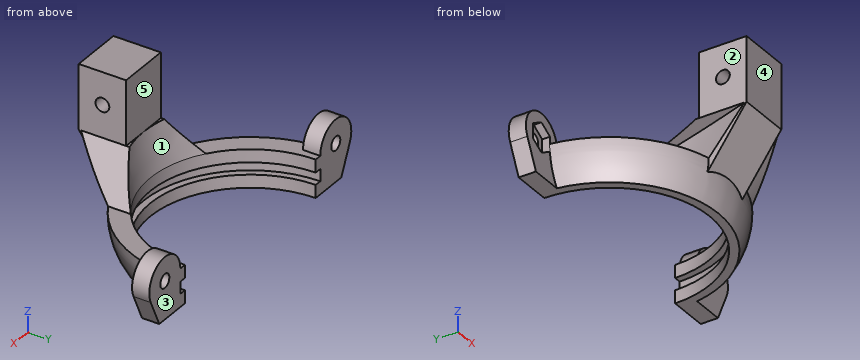
```python
from build123d import *

# Parameters (mm, degrees)
SKETCH005_R          = 1.6
PAD001_DEPTH         = 6.15
REVOLUTION_ANGLE     = -180
PAD_DEPTH            = 4
SKETCH002_R          = 1.6
POCKET_DEPTH         = 5
POCKET001_DEPTH      = 1.8
SKETCH004_R          = 3
POCKET002_DEPTH      = 2
REVOLUTION001_ANGLE  = 70
POCKET003_DEPTH      = 184.719613
POCKET003_DEPTH_BACK = 198.519612


with BuildPart() as pad001:
    # Sketch005 → Pad001 (new body, symmetric)
    with BuildSketch(Plane.YZ):
        Polygon((-35.8, 27.909628), (-24.8, 27.909628), (-24.8, -2.8), (-35.8, 12.909628), align=None)
        with Locations((-30.3, 20.409628)):
            Circle(SKETCH005_R, mode=Mode.SUBTRACT)
    extrude(amount=PAD001_DEPTH, both=True)


with BuildPart() as obj1:
    # Sketch → Revolution (revolve)
    with BuildSketch(Plane.XZ):
        with BuildLine():
            Line((23.2, 0), (24.8, 0))
            Line((24.8, 0), (24.8, -2.8))
            Line((24.8, -2.8), (23.2, -2.8))
            Line((23.2, -2.8), (23.2, -5.8))
            Line((23.2, -5.8), (25.2, -5.8))
            ThreePointArc((25.2, -5.8), (27.062874, -1.574112), (27.7, 3))
            Line((27.7, 3), (23.2, 3))
            Line((23.2, 0), (23.2, 3))
        make_face()
    revolve(axis=Axis((0, 0, 0), (0, 0, 1)), revolution_arc=REVOLUTION_ANGLE)

    # Sketch001 → Pad (new body)
    with BuildSketch(Plane(origin=(0, 0, 0), x_dir=(1, 0, 0), z_dir=(0, 1, 0))):
        with BuildLine():
            ThreePointArc((24.8, -3), (31.490407, -8.36963), (35.284703, -0.67562))
            Line((32.265071, 5.8), (35.284703, -0.67562))
            Line((24.8, 5.8), (32.265071, 5.8))
            Line((24.8, -3), (24.8, 5.8))
        make_face()
    pad = extrude(amount=-PAD_DEPTH)

    # Mirrored: Pad across Sketch001 V_Axis
    add(pad.mirror(Plane.YZ))

    # Sketch002 → Pocket (cut)
    with BuildSketch(Plane(origin=(0, 0, 0), x_dir=(1, 0, 0), z_dir=(0, 1, 0))):
        with Locations((-30.3, -3)):
            Circle(SKETCH002_R)
    pocket = extrude(amount=-POCKET_DEPTH, mode=Mode.SUBTRACT)

    # Mirrored001: Pocket across Sketch002 V_Axis
    add(pocket.mirror(Plane.YZ), mode=Mode.SUBTRACT)

    # Sketch003 → Pocket001 (cut)
    with BuildSketch(Plane.XZ.offset(4)):
        Polygon((-30.3, 6.464101), (-33.3, 4.73205), (-33.3, 1.267949), (-30.3, -0.464102), (-27.3, 1.267949), (-27.3, 4.73205), align=None)
    extrude(amount=-POCKET001_DEPTH, mode=Mode.SUBTRACT)

    # Sketch004 → Pocket002 (cut)
    with BuildSketch(Plane.XZ.offset(4)):
        with Locations((30.3, 3)):
            Circle(SKETCH004_R)
    extrude(amount=POCKET002_DEPTH, mode=Mode.SUBTRACT)

    # Fusion: union Pad001
    add(pad001.part)


with BuildPart() as mount_part:
    # Sketch006 → Revolution001 (revolve, symmetric)
    with BuildSketch(Plane.YZ) as revolution001_sk:
        Polygon((-23.2, 3), (-27.7, 3), (-35.8, 12.909628), (-24.8, 12.909628), align=None)
    revolve(axis=Axis((0, 0, 0), (0, 0, 1)), revolution_arc=REVOLUTION001_ANGLE / 2)
    revolve(revolution001_sk.sketch, axis=Axis((0, 0, 0), (0, 0, -1)), revolution_arc=REVOLUTION001_ANGLE / 2)

    # Fusion001: union obj1
    add(obj1.part)

    # Sketch007 → Pocket003 (cut, two sides)
    with BuildSketch(Plane(origin=(0, -24.8, 0), x_dir=(-1, 0, 0), z_dir=(0, 1, 0))) as pocket003_sk:
        Polygon((-15.888067, 3), (-13.306973, 3), (-6.15, 12.909628), (-29.113317, 25.73584), align=None)
    pocket003 = extrude(amount=-POCKET003_DEPTH, mode=Mode.SUBTRACT) + extrude(pocket003_sk.sketch, amount=POCKET003_DEPTH_BACK, mode=Mode.SUBTRACT)

    # Mirrored002: Pocket003 across Sketch007 V_Axis
    add(pocket003.mirror(Plane(origin=(0, -24.8, 0), x_dir=(0, 1, 0), z_dir=(-1, 0, 0))), mode=Mode.SUBTRACT)


solid = mount_part.part
```
Part model, mm, in its own coordinate system. Face numbers are marked on the shaded views. A direction names the side the tool comes from. Coordinates: 2 decimals unless noted, no trailing zeros. Write each loop counter-clockwise with the first axis right and the second up, starting at its lowest first coordinate (ties: lowest second). Pieces come first, ordered by that corner, then holes.
Item 1: Which spindle directions (+Z, -Z, +X, -X, +Y, -Y) get a long thin tool onto all of the face, cutting with end or side? Do the marked faces 4 and 5. Say none if no direction does.
Item 2: Slice it at C-C (z = 15). Write the cut outline in (x, y), and give its area (3 significant figures).
Item 3: Mould opens along X. For the marked faces 1, 2 and 3 say: released by +X, released by -X, zero draft, split by the parting line, or undercut.
Item 4: Pin check, flat tips, straight feed: pin 1 (3.5 mm diameter, centred on x = 2, z = 18.5, fed in from +Y); pin 2 (1.5 mm diameter, centred on y = -24, z = -0.5, fed in from -X); pin 3 (0.5 mm diameter, centred on y = -3, z = 2.5, fed in from +X). Stop position of each tip, or through.
Item 5: Probe line 1 (Z direction, x = -30.3, y = -0.75); line 2 (Z direction, x = -1.5, y = -30.3); line 3 (X direction, y = -26, z = 27.5). List the from-to ranges inside material, lowest first.
Item 6: Slice it at A-A (x = 30.3). Write the cut outline in (y, z), and give its area (3 significant figures).
Item 7: Slice it at B-B (z = 11.5). Write the cut outline in (x, y).
Results found:
1. face 4: +Z, -Z, +X, -X, -Y
1. face 5: +Z, +X, -X, +Y
2. outline: (-6.15, -35.8) - (6.15, -35.8) - (6.15, -24.8) - (-6.15, -24.8) - close
2. area: 135 mm2
3. face 1: undercut
3. face 2: released by -X
3. face 3: zero draft
4. pin 1: stops at y = -24.8
4. pin 2: stops at x = -14.4
4. pin 3: stops at x = 35.79
5. line 1: z = -5.8 to 1.4, 4.6 to 8.5
5. line 2: z = 5.05 to 18.81, 22.01 to 27.91
5. line 3: x = -6.15 to 6.15
6. outline: (-4, -5.8) - (0, -5.8) - (0, 1.4) - (-4, 1.4) - close; (-4, 4.6) - (0, 4.6) - (0, 8.5) - (-4, 8.5) - close
6. area: 44.4 mm2
7. outline: (-7.17, -33.9) arc R34.65 ccw to (-6.15, -34.1) - (-6.15, -34.81) - (6.15, -34.81) - (6.15, -34.1) arc R34.65 ccw to (7.17, -33.9) - (7.17, -23.5) arc R24.57 cw to (-7.17, -23.5) - close
